```python
from build123d import *

# Parameters (mm, degrees)
SKETCH1_W           = 17.2
SKETCH1_H           = 10.85
BOSS_EXTRUDE1_DEPTH = 1.65
SKETCH2_R           = 4.85
BOSS_EXTRUDE2_DEPTH = 4.75
FILLET1_R           = 0.5
SKETCH3_W           = 1.359488803
SKETCH3_H           = 3.031292602
SKETCH3_W_2         = 1.800404091
SKETCH3_H_2         = 0.955316456
SKETCH3_W_3         = 0.863459105
SKETCH3_H_3         = 1.72691821
SKETCH3_W_4         = 0.918573516
SKETCH3_W_5         = 1.910632913
SKETCH3_H_4         = 0.936944986
SKETCH3_H_5         = 0.973687927
SKETCH3_W_6         = 2.020861734
SKETCH3_W_7         = 0.936944986
SKETCH3_H_6         = 2.112719086
SKETCH3_W_8         = 1.855518501
SKETCH3_H_7         = 0.992059397
BOSS_EXTRUDE3_DEPTH = 1


with BuildPart() as part:
    # Sketch1 → Boss-Extrude1 (new body)
    with BuildSketch(Plane(origin=(0, 0, 0), x_dir=(1, 0, 0), z_dir=(0, 1, 0))):
        Rectangle(SKETCH1_W, SKETCH1_H)
    extrude(amount=BOSS_EXTRUDE1_DEPTH)

    # Sketch2 → Boss-Extrude2 (add)
    with BuildSketch(Plane(origin=(0, 1.65, 0), x_dir=(1, 0, 0), z_dir=(0, 1, 0))):
        with Locations((3.75, 0)):
            Circle(SKETCH2_R)
    extrude(amount=BOSS_EXTRUDE2_DEPTH)

    # Fillet1
    fillet1_edges = [part.edges().sort_by_distance(p)[0] for p in [
        (-1.1, 6.4, 0),
    ]]
    fillet(fillet1_edges, radius=FILLET1_R)

    # Sketch3 → Boss-Extrude3 (add)
    with BuildSketch(Plane.XZ):
        with Locations((-0.679744402, -0.192900438)):
            Rectangle(SKETCH3_W, SKETCH3_H)
        with Locations((-0.624629991, -2.755720547)):
            Rectangle(SKETCH3_W_2, SKETCH3_H_2)
        with Locations((-3.554879506, 0.055114411)):
            Rectangle(SKETCH3_W_3, SKETCH3_H_3)
        with Locations((-4.997039925, 0.055114411)):
            Rectangle(SKETCH3_W_4, SKETCH3_H_3)
        with Locations((-0.679744402, 3.995794793)):
            Rectangle(SKETCH3_W_5, SKETCH3_H_4)
        with Locations((-0.679744402, 2.746534812)):
            Rectangle(SKETCH3_W_5, SKETCH3_H_5)
        with Locations((3.159892894, 4.197880967)):
            Rectangle(SKETCH3_W_6, SKETCH3_H_5)
        with Locations((2.103533351, 1.46053189)):
            Rectangle(SKETCH3_W_7, SKETCH3_H_6)
        with Locations((3.398722008, 1.46053189)):
            Rectangle(SKETCH3_W_4, SKETCH3_H_6)
        with Locations((3.077221278, -1.414603215)):
            Rectangle(SKETCH3_W_8, SKETCH3_H_7)
    extrude(amount=BOSS_EXTRUDE3_DEPTH)


solid = part.part
```
Check sheet for the modelled part. Datum: model origin and axes. Units: mm. A direction names the side the tool comes from. Round coordinates to 2 decimals unless told otherwise and drop trailing zeros. Order: outer loops, then holes, each group sorted by start corner. A loop starts at its lowest first (then second) coordinate and runs counter-clockwise, first axis right, second up. Notation, with made-up numbers: (-38.5, 8.25) -> (-27.5, 8.25) arc R25 cw to (-27.5, 27.25) -> close; hole circle Ø11 at (-16.5, 35.5). An arc over 180 degrees is marked (long way). One line per item, written item: value. Start each with the question number.
Q1. Set-up check for faces 1 (the face through (-1.635, -0.5, 2.7)), 2 (the face through (3.4, -0.5, 2.517)), 3 (the face through (3.1, -0.5, -1.911)): record each of +Z, -Z, +X, -X, +Y, -Y from which the full face is reachable in a straight line by a thin tool's end or side.
Q2. Mould release check, pull along Z, two halves, no side actions. Record for faces 4 (the face through (3.858, -0.5, 1.4)), 5 (the face through (2.572, -0.5, 1.4)), 6 (the face through (3.1, -1, -1.4)), 7 (the face through (-5, -0.5, -0.808)): pulls with the +Z half, pulls with the -Z half, needs draft (parallel to the pull), parting line crosses it, or undercut.
Q3. Thickness scan on line 1 (Y direction, x = 7.5, z = 0.75); line 2 (Y direction, x = -6.75, z = 2.5); line 3 (X direction, y = 5, z = 1.25). Record the ranges inside material, lowest first.
Q4. Gauge pin test, flat ends, axial feed: pin 1 Ø0.7 at (x, y) = (-3.5, -0.5) entering from -Z; pin 2 Ø0.5 at (y, z) = (-0.5, 4) entering from -X; pin 3 Ø1.1 at (y, z) = (-0.5, -2.5) entering from -X; pin 4 Ø0.5 at (x, y) = (-1, -0.5) entering from +Z. Record the tip position at first contact, or that the pin passes through.
Q5. Cross-section at B-B (x = -4.25). Record the boundary of the cut face in (y, z) (3 decimals), and give its area (3 significant figures).
Q6. Cross-section at A-A (y = 5.25). Record the boundary of the cut face in (x, z), and give its area (3 significant figures).
Completed:
1. face 1: +Z, -Z, -X, -Y
1. face 2: +X, -Y
1. face 3: -Z, +X, -X, -Y
2. face 4: undercut
2. face 5: undercut
2. face 6: needs draft
2. face 7: pulls with the -Z half
3. line 1: y = 0 to 6.4
3. line 2: y = 0 to 1.65
3. line 3: x = -0.94 to 8.44
4. pin 1: stops at z = -0.81
4. pin 2: stops at x = -1.64
4. pin 3: stops at x = -8.6
4. pin 4: stops at z = 4.46
5. outline: (0, -5.425) -> (1.65, -5.425) -> (1.65, 5.425) -> (0, 5.425) -> close
5. area: 17.9 mm²
6. outline: circle Ø9.7 at (3.75, 0)
6. area: 73.9 mm²
